from build123d import *

# Parameters (mm, degrees)
BOSS_EXTRUDE1_DEPTH = 31.75
SKETCH19_W          = 15.860402013
SKETCH19_H          = 31.75
BOSS_EXTRUDE7_DEPTH = 2
SKETCH23_W          = 15.860402013
SKETCH23_H          = 1
BOSS_EXTRUDE8_DEPTH = 25
SKETCH24_R          = 1.27
CUT_EXTRUDE1_DEPTH  = 2.54


with BuildPart() as part:
    # Sketch2 → Boss-Extrude1 (new body)
    with BuildSketch(Plane.XY):
        with BuildLine():
            Line((-50.375618534, 45.609862895), (-50.351188886, 46.309436474))
            ThreePointArc((-50.351188886, 46.309436474), (-50.565618587, 46.88295476), (-51.12278195, 47.136868733))
            Line((-51.12278195, 47.136868733), (-55.780902554, 47.299533889))
            Line((-55.780902554, 47.299533889), (-47.850701548, 47.299533889))
            Line((-47.850701548, 47.299533889), (-47.850701548, 40.900752235))
            Line((-47.850701548, 40.900752235), (-48.952946324, 40.900752235))
            ThreePointArc((-48.952946324, 40.900752235), (-50.100996621, 41.129113637), (-51.074266668, 41.779431891))
            Line((-51.074266668, 41.779431891), (-53.375146928, 44.080312152))
            ThreePointArc((-53.375146928, 44.080312152), (-53.536830204, 44.931922499), (-52.803734096, 45.394471696))
            Line((-52.803734096, 45.394471696), (-50.685905631, 45.320515496))
            ThreePointArc((-50.685905631, 45.320515496), (-50.470836274, 45.400926634), (-50.375618534, 45.609862895))
        make_face()
    boss_extrude1 = extrude(amount=BOSS_EXTRUDE1_DEPTH)

    # Mirror2: Boss-Extrude1 across plane
    add(boss_extrude1.mirror(Plane(origin=(-47.850701548, 40.900752235, 31.75), x_dir=(0, 0, 1), z_dir=(-1, 0, 0))))

    # Sketch19 → Boss-Extrude7 (add)
    with BuildSketch(Plane(origin=(0, 47.299533889, 0), x_dir=(1, 0, 0), z_dir=(0, 1, 0))):
        with Locations((-47.850701548, -15.875)):
            Rectangle(SKETCH19_W, SKETCH19_H)
    extrude(amount=BOSS_EXTRUDE7_DEPTH)

    # Sketch23 → Boss-Extrude8 (add)
    with BuildSketch(Plane(origin=(0, 49.299533889, 0), x_dir=(1, 0, 0), z_dir=(0, 1, 0))):
        with Locations((-47.850701548, -31.25)):
            Rectangle(SKETCH23_W, SKETCH23_H)
    extrude(amount=BOSS_EXTRUDE8_DEPTH)

    # Sketch24 → Cut-Extrude1 (cut)
    with BuildSketch(Plane(origin=(0, 0, 30.75), x_dir=(-1, 0, 0), z_dir=(0, 0, -1))):
        with Locations((47.850701548, 67.949533889)):
            Circle(SKETCH24_R)
    extrude(amount=-CUT_EXTRUDE1_DEPTH, mode=Mode.SUBTRACT)


solid = part.part
Verification items for the finished model (mm, model axes). A direction names the side the tool comes from. Round coordinates to 2 decimals unless told otherwise and drop trailing zeros. Loops run counter-clockwise (first coordinate to the right, second up) from the corner with the lowest first, then second, coordinate; pieces in that order, holes last. Notation, with made-up numbers: (-15.75, -36) - (31.25, -36) arc R27 cw to (31.25, 0) - close; hole circle Ø4 at (11.5, 35). An arc over 180 degrees is marked (long way). Use one line per item in the form item = value.
1. Access from +Z, -Z, +X, -X, +Y, -Y to the whole of each face (thin tool, end or side, straight path). Record for faces 1 (the cylindrical face through (-50.56, 46.876, 15.653)), 2 (the flat face through (-48, 49.3, 15)), 3 (the flat face through (-43.493, 42.914, 15.653)).
A:
face_1 = +Z, -Z, -X
face_2 = -Z, +X, -X, +Y
face_3 = +Z, -Z, +X, -Y
2. Section check B-B on z = 3. Record the cut outline in (x, y), and give its area (3 significant figures).
A:
outline = (-55.78, 47.3) - (-51.12, 47.14) arc R0.8 cw to (-50.35, 46.31) - (-50.38, 45.61) arc R0.3 cw to (-50.69, 45.32) - (-52.8, 45.39) arc R0.77 ccw to (-53.38, 44.08) - (-51.07, 41.78) arc R3 ccw to (-48.95, 40.9) - (-46.75, 40.9) arc R3 ccw to (-44.63, 41.78) - (-42.33, 44.08) arc R0.77 ccw to (-42.9, 45.39) - (-45.02, 45.32) arc R0.3 cw to (-45.33, 45.61) - (-45.35, 46.31) arc R0.8 cw to (-44.58, 47.14) - (-39.92, 47.3) - (-39.92, 49.3) - (-55.78, 49.3) - close
area = 81.8 mm²
3. Section check A-A on x = -43.5. Record the cut outline in (y, z).
A:
outline = (42.91, 0) - (45.37, 0) - (45.37, 31.75) - (42.91, 31.75) - close; (47.17, 0) - (49.3, 0) - (49.3, 30.75) - (74.3, 30.75) - (74.3, 31.75) - (47.17, 31.75) - close
4. Gauge pin test, flat ends, axial feed: pin 1 Ø8 at (x, y) = (-47, 64.5) entering from -Z; pin 2 Ø1.5 at (x, z) = (-42.5, 21.5) entering from +Y. Record the tip position at first contact, or that the pin passes through.
A:
pin_1 = 30.75
pin_2 = 49.3
5. Draft check along Y on faces 4 (the cylindrical face through (-45, 47, 16)), 5 (the flat face through (-48, 62, 30.75)), 6 (the flat face through (-52.209, 42.914, 15.653)). Enter one of: pulls with the +Y half, pulls with the -Y half, needs draft (parallel to the pull), parting line crosses it, or undercut.
A:
face_4 = undercut
face_5 = needs draft
face_6 = pulls with the -Y half
6. Section check C-C on y = 62.5. Record the cut outline in (x, z).
A:
outline = (-55.78, 30.75) - (-39.92, 30.75) - (-39.92, 31.75) - (-55.78, 31.75) - close
7. Scan lines: probe 1 along Y at (x, z) = (-48, 19); probe 2 along Z at (x, y) = (-43.5, 66.5); probe 3 along Y at (x, z) = (-51, 30). Record each from-to range of solid material in increasing order.
A:
probe_1 = 40.9 to 49.3
probe_2 = 30.75 to 31.75
probe_3 = 41.71 to 45.33, 47.12 to 49.3
